```python
from build123d import *

# Parameters (mm, degrees)
F1_DEPTH = 10


with BuildPart() as f1:
    # F0 (on Top) → F1 (new body)
    with BuildSketch(Plane.XY):
        with BuildLine():
            Line((-4, 0), (0, 0))
            Line((0, 0), (0, 10))
            Line((0, 10), (14.4, 10))
            Line((14.4, 10), (14.4, -50))
            ThreePointArc((14.4, -50), (24.4, -60), (34.4, -50))
            ThreePointArc((34.4, -50), (32.4, -48), (30.4, -50))
            ThreePointArc((30.4, -50), (24.4, -56), (18.4, -50))
            Line((18.4, -50), (18.4, 14))
            Line((18.4, 14), (-4, 14))
            Line((-4, 14), (-4, 0))
        make_face()
    extrude(amount=F1_DEPTH)


solid = f1.part
```
The listing builds one solid part. Answer for the finished solid, in the listing's coordinates (mm). A direction names the side the tool comes from. Coordinates: 2 decimals unless noted, no trailing zeros. Loops run counter-clockwise (first coordinate to the right, second up) from the corner with the lowest first, then second, coordinate; pieces in that order, holes last. Notation, with made-up numbers: M -14.75,86.25 L -9.75,86.25 A19 ccw -9.75,93.25 Z; hole C 73,79.5 d9. An arc over 180 degrees is marked long. Answer as a JSON object with one key per item and string values. Group by question number.
Item 1: Section D-D (y = -7) is taken. Write down the section's boundary in (x, z).
Item 2: Determine the mould class of faces 1 (the face through (14.4, -20, 5)), 2 (the face through (24.5, -56, 4.9)), 3 (the face through (15, -20, 10)), 4 (the face through (24.2, -60, 4.9)) for opening direction X: +X half, -X half, draft (parallel to the pull), parting line (faces both ways), or undercut.
Item 3: Section B-B (z = 6.25) is taken. Write down the section's boundary in (x, y), and give its area (3 significant figures).
Item 4: Which of the six approach directions +Z, -Z, +X, -X, +Y, -Y give full straight-line access (tool end or side, diameter ignored) to faces 5 (the face through (-2, 0, 5)), 6 (the face through (7, 14, 5)), 7 (the face through (7, 10, 5))?
Item 5: Section A-A (y = 8.5) is taken. Write down the section's boundary in (x, z).
Item 6: Consider L1, parallel to X at y = 5.5, z = 5; L2, parallel to X at y = -38, z = 8.75; L3, parallel to X at y = -55, z = 9.25. Determine where each line is inside the solid, lowest interval first.
Item 7: Section C-C (x = 32.4) is taken. Write down the section's boundary in (y, z), and give its area (3 significant figures).
Item 8: Each of these flat-tipped pins is pushed along its axis until it touches: P1, Ø3, axis at y = -7.5, z = 4, coming from the +X side; P2, Ø4, axis at x = 25.5, z = 6, coming from the +Y side; P3, Ø2, axis at y = -29, z = 2.5, coming from the -X side. Where does it stop, or does it pass through?
Solved:
{
 "1": {"outline": "M 14.4,0 L 18.4,0 L 18.4,10 L 14.4,10 Z"},
 "2": {"face 1": "undercut", "face 2": "undercut", "face 3": "draft", "face 4": "parting line"},
 "3": {"outline": "M -4,0 L 0,0 L 0,10 L 14.4,10 L 14.4,-50 A10 ccw 34.4,-50 A2 ccw 30.4,-50 A6 cw 18.4,-50 L 18.4,14 L -4,14 Z", "area": "476 mm2"},
 "4": {"face 5": "+Z, -Z, -X, -Y", "face 6": "+Z, -Z, +X, -X, +Y", "face 7": "+Z, -Z, -Y"},
 "5": {"outline": "M -4,0 L 0,0 L 0,10 L -4,10 Z; M 14.4,0 L 18.4,0 L 18.4,10 L 14.4,10 Z"},
 "6": {"L1": "x = -4 to 0, 14.4 to 18.4", "L2": "x = 14.4 to 18.4", "L3": "x = 15.74 to 21.08, 27.72 to 33.06"},
 "7": {"outline": "M -56,0 L -48,0 L -48,10 L -56,10 Z", "area": "80.0 mm2"},
 "8": {"P1": "stops at x = 18.4", "P2": "stops at y = -55.14", "P3": "stops at x = 14.4"}
}
